The model under review builds one solid part; all positions refer to its coordinate system, in mm. Give positions to 0.01 mm unless a question says otherwise; leave off trailing zeros. Order: outer loops, then holes, each group sorted by start corner. A loop starts at its lowest first (then second) coordinate and runs counter-clockwise, first axis right, second up. Notation, with made-up numbers: (-23.5, 61) - (18.5, 61) arc R27 ccw to (18.5, 84) - close; hole circle Ø5 at (-9, 17). An arc over 180 degrees is marked (long way). Write item = value, one per line. Start each with the question number.
1. Wall thickness on probe 1 along Z at (x, y) = (0.4, 2.25); probe 2 along Y at (x, z) = (0.1, -8); probe 3 along Z at (x, y) = (0.3, 3.5): over which ranges is each line inside the solid? List them lowest first.
2. We need section C-C, the plane z = -8. Give the boundary of the cut face in (x, y), and give its area (3 significant figures).
3. We need section D-D, the plane z = -28. Give the boundary of the cut face in (x, y), and give its area (3 significant figures).
4. Mouldability with a two-part tool opening along X and no side actions: class faces 1 (the flat face through (0.5, 10, -34)), 2 (the flat face through (0, 0, -28)), 3 (the flat face through (-0.5, 10, -34)) as pulls with the +X half, pulls with the -X half, needs draft (parallel to the pull), parting line crosses it, or undercut.
5. We need section B-B, the plane x = 0. Give the boundary of the cut face in (y, z).
6. We need section A-A, the plane y = 4.5. Give the boundary of the cut face in (x, z).
from build123d import *

# Parameters (mm, degrees)
BOSS_EXTRUDE1_DEPTH      = 0.5
BOSS_EXTRUDE1_DEPTH_BACK = 0.5
FILLET1_R                = 1
SKETCH2_R                = 2.75
CUT_EXTRUDE1_DEPTH       = 60.661042565


with BuildPart() as part:
    # Sketch1 → Boss-Extrude1 (new, two sides: drawn at the far end of the back side and taken through both)
    with BuildSketch(Plane(origin=(0, 0, 0), x_dir=(0, 0, -1), z_dir=(1, 0, 0)).offset(-BOSS_EXTRUDE1_DEPTH_BACK)):
        Polygon((0, 0), (56.2, 0), (56.2, 20), (36.2, 20), (0, 9), align=None)
    extrude(amount=BOSS_EXTRUDE1_DEPTH + BOSS_EXTRUDE1_DEPTH_BACK)

    # Fillet1
    fillet1_edges = [part.edges().sort_by_distance(p)[0] for p in [
        (0, 9, 0),
        (0, 20, -36.2),
        (0, 20, -56.2),
        (0, 0, -56.2),
        (0, 0, 0),
    ]]
    fillet(fillet1_edges, radius=FILLET1_R)

    # Sketch2 → Cut-Extrude1 (cut, through all)
    with BuildSketch(Plane(origin=(0.5, 0, 0), x_dir=(0, 0, -1), z_dir=(1, 0, 0))):
        with Locations((8, 4.5)):
            Circle(SKETCH2_R)
        with Locations((28, 4.5)):
            Circle(SKETCH2_R)
    extrude(amount=-CUT_EXTRUDE1_DEPTH, mode=Mode.SUBTRACT)


solid = part.part
Model answer:
q1.probe_1 = -56.2 to -29.58, -26.42 to -9.58, -6.42 to 0
q1.probe_2 = 0 to 1.75, 7.25 to 11.43
q1.probe_3 = -56.2 to -30.56, -25.44 to -10.56, -5.44 to 0
q2.outline = (-0.5, 0) - (0.5, 0) - (0.5, 1.75) - (-0.5, 1.75) - close; (-0.5, 7.25) - (0.5, 7.25) - (0.5, 11.43) - (-0.5, 11.43) - close
q2.area = 5.93 mm2
q3.outline = (-0.5, 0) - (0.5, 0) - (0.5, 1.75) - (-0.5, 1.75) - close; (-0.5, 7.25) - (0.5, 7.25) - (0.5, 17.51) - (-0.5, 17.51) - close
q3.area = 12.0 mm2
q4.face_1 = pulls with the +X half
q4.face_2 = needs draft
q4.face_3 = pulls with the -X half
q5.outline = (0, -55.2) arc R1 ccw to (1, -56.2) - (19, -56.2) arc R1 ccw to (20, -55.2) - (20, -36.35) arc R1 ccw to (19.96, -36.06) - (9.22, -0.71) arc R1 ccw to (8.26, 0) - (1, 0) arc R1 ccw to (0, -1) - close; hole circle Ø5.5 at (4.5, -28); hole circle Ø5.5 at (4.5, -8)
q6.outline = (-0.5, -56.2) - (0.5, -56.2) - (0.5, -30.75) - (-0.5, -30.75) - close; (-0.5, -25.25) - (0.5, -25.25) - (0.5, -10.75) - (-0.5, -10.75) - close; (-0.5, -5.25) - (0.5, -5.25) - (0.5, 0) - (-0.5, 0) - close
